Geometry: see drawing. Coordinates: mm, zero at the bounding-box minimum. A direction names the side the tool comes from. Give positions to 0.01 mm unless a question says otherwise; leave off trailing zeros. Order: outer loops, then holes, each group sorted by start corner. A loop starts at its lowest first (then second) coordinate and runs counter-clockwise, first axis right, second up. Notation, with made-up numbers: M -21.5,9 L 6.5,9 A17 cw 6.5,25 Z; hole C -5,83.5 d1. An arc over 180 degrees is marked long. Use a Markdown table: item, result.
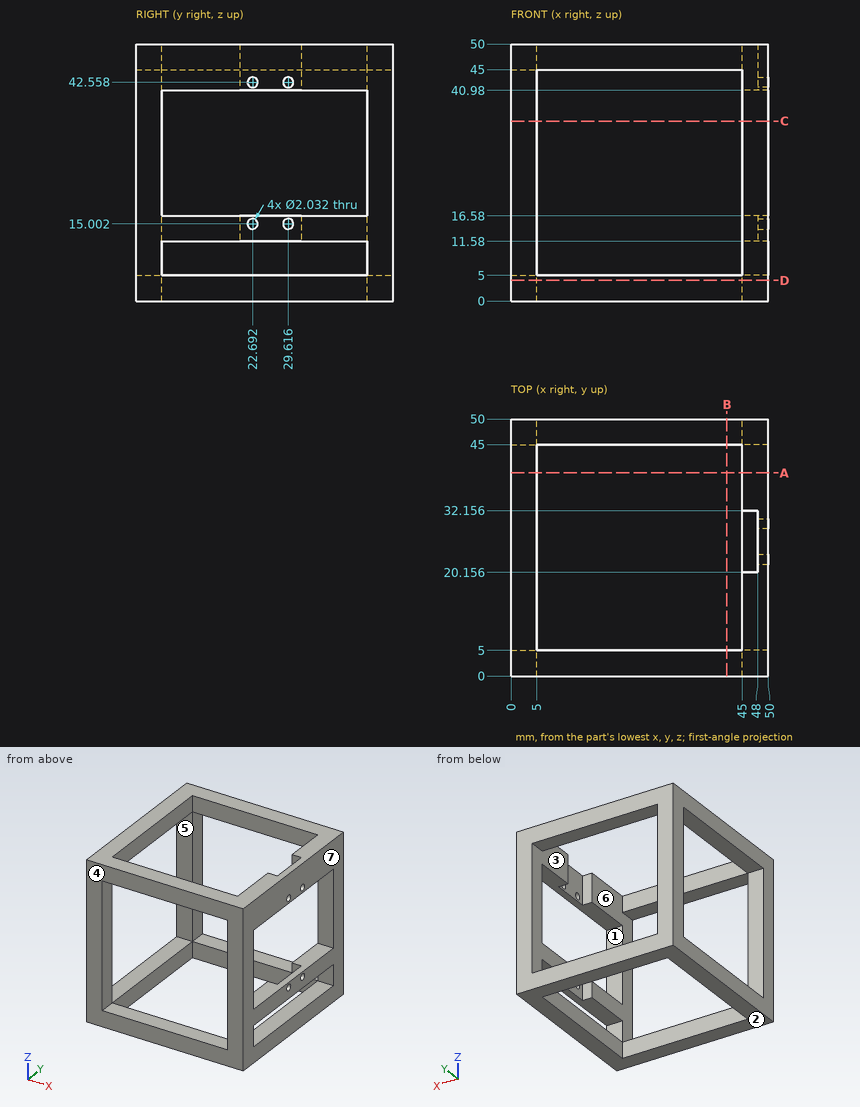
1) Cut plane A-A on y = 39.5. Return loops of the section in (x, z).
Response values:
| item | result |
|---|---|
| outline | M 0,0 L 5,0 L 5,5 L 0,5 Z; M 0,45 L 5,45 L 5,50 L 0,50 Z; M 45,0 L 50,0 L 50,5 L 45,5 Z; M 45,11.58 L 50,11.58 L 50,16.58 L 45,16.58 Z; M 45,40.98 L 50,40.98 L 50,50 L 45,50 Z |
2) First-contact query: pin 1 Ø1.5 at (y, z) = (32, 13.5) entering from -X. Flat tip, straight axial feed; report the tip coordinate or a pass-through.
Response values:
| item | result |
|---|---|
| pin 1 | stops at x = 45 |
3) Cut plane B-B on x = 42. Return loops of the section in (y, z).
Response values:
| item | result |
|---|---|
| outline | M 0,0 L 5,0 L 5,5 L 0,5 Z; M 0,45 L 5,45 L 5,50 L 0,50 Z; M 45,0 L 50,0 L 50,5 L 45,5 Z; M 45,45 L 50,45 L 50,50 L 45,50 Z |
4) Material intervals for line 1 (Z direction, x = 45.5, y = 10); line 2 (Y direction, x = 46, z = 45); line 3 (X direction, y = 6, z = 47), sorted ascending. Write a range as from..to.
Response values:
| item | result |
|---|---|
| line 1 | z = 0..5, 11.58..16.58, 40.98..50 |
| line 2 | y = 0..20.16, 32.16..50 |
| line 3 | x = 0..5, 45..50 |
5) Mould query, pull axis Y, two halves, no side actions, for the marked faces 4, 5, 6 and 7. Classes: released by +Y, released by -Y, zero draft, split by the parting line, or undercut.
Response values:
| item | result |
|---|---|
| face 4 | released by -Y |
| face 5 | undercut |
| face 6 | undercut |
| face 7 | zero draft |
6) Cut plane D-D on z = 4. Return loops of the section in (x, y), and give its area (3 significant figures).
Response values:
| item | result |
|---|---|
| outline | M 0,0 L 50,0 L 50,50 L 0,50 Z; hole M 5,5 L 45,5 L 45,45 L 5,45 Z |
| area | 900 mm² |
7) Reachability of the marked faces 1, 2 and 3 from +Z, -Z, +X, -X, +Y, -Y: full face, straight path, thin tool, end or side. Return the list, or none.
Response values:
| item | result |
|---|---|
| face 1 | +X, -X |
| face 2 | -Z, +X, -X, +Y, -Y |
| face 3 | none |
